Part model, mm, in its own coordinate system. A direction names the side the tool comes from. Round coordinates to 2 decimals unless told otherwise and drop trailing zeros. Order: outer loops, then holes, each group sorted by start corner. A loop starts at its lowest first (then second) coordinate and runs counter-clockwise, first axis right, second up. Notation, with made-up numbers: (66, 35) - (92, 35) arc R16 ccw to (92, 46) - close; hole circle Ø3 at (89, 71.5). An arc over 180 degrees is marked (long way). Answer as a JSON object with one key per item and string values.
```python
from build123d import *

# Parameters (mm, degrees)
SKETCH1_R           = 37.5
SKETCH1_R_2         = 27.5
BOSS_EXTRUDE1_DEPTH = 15
SKETCH2_R           = 32.5
SKETCH2_R_2         = 27.5
CUT_EXTRUDE1_DEPTH  = 7
SKETCH3_W           = 5
SKETCH3_H           = 40
CUT_EXTRUDE2_DEPTH  = 45
BOSS_EXTRUDE2_DEPTH = 45
SKETCH6_W           = 10
SKETCH6_H           = 40
CUT_EXTRUDE3_DEPTH  = 5
SKETCH7_W           = 10
SKETCH7_H           = 40
BOSS_EXTRUDE3_DEPTH = 12.5
SKETCH8_R           = 1.5
CUT_EXTRUDE4_DEPTH  = 10


with BuildPart() as part:
    # Sketch1 → Boss-Extrude1 (new body)
    # profile 1 of 2: a face of its own
    with BuildSketch(Plane.XY):
        Circle(SKETCH1_R)
        Circle(SKETCH1_R_2, mode=Mode.SUBTRACT)
    # profile 2 of 2: a face of its own
    with BuildSketch(Plane.XY):
        with BuildLine():
            Line((-23.101603537, -77.5), (21.898396463, -77.5))
            Line((21.898396463, -77.5), (21.898396463, -30.441915714))
            ThreePointArc((21.898396463, -30.441915714), (-0.752089542, -37.492457392), (-23.101603537, -29.5392267))
            Line((-23.101603537, -29.5392267), (-23.101603537, -77.5))
        make_face()
    extrude(amount=BOSS_EXTRUDE1_DEPTH)

    # Sketch2 → Cut-Extrude1 (cut)
    with BuildSketch(Plane(origin=(0, 0, 0), x_dir=(-1, 0, 0), z_dir=(0, 0, -1))):
        Circle(SKETCH2_R)
        Circle(SKETCH2_R_2, mode=Mode.SUBTRACT)
    extrude(amount=-CUT_EXTRUDE1_DEPTH, mode=Mode.SUBTRACT)

    # Sketch3 → Cut-Extrude2 (cut)
    with BuildSketch(Plane(origin=(21.898396463, 0, 0), x_dir=(0, 0, -1), z_dir=(1, 0, 0))):
        with Locations((-12.5, -57.5)):
            Rectangle(SKETCH3_W, SKETCH3_H)
    extrude(amount=-CUT_EXTRUDE2_DEPTH, mode=Mode.SUBTRACT)

    # Sketch5 → Boss-Extrude2 (add)
    with BuildSketch(Plane.ZY.offset(23.101603537)):
        Polygon((10, -37.5), (15, -37.5), (10, -77.5), align=None)
    extrude(amount=-BOSS_EXTRUDE2_DEPTH)

    # Sketch6 → Cut-Extrude3 (cut)
    with BuildSketch(Plane.XY.offset(15)):
        with Locations((-10.101603537, -57.5)):
            Rectangle(SKETCH6_W, SKETCH6_H)
        with Locations((8.898396463, -57.5)):
            Rectangle(SKETCH6_W, SKETCH6_H)
    extrude(amount=-CUT_EXTRUDE3_DEPTH, mode=Mode.SUBTRACT)

    # Sketch7 → Boss-Extrude3 (add)
    with BuildSketch(Plane(origin=(0, 0, 0), x_dir=(-1, 0, 0), z_dir=(0, 0, -1))):
        with Locations((-16.898396463, -57.5)):
            Rectangle(SKETCH7_W, SKETCH7_H)
        with Locations((18.101603537, -57.5)):
            Rectangle(SKETCH7_W, SKETCH7_H)
    extrude(amount=BOSS_EXTRUDE3_DEPTH)

    # Sketch8 → Cut-Extrude4 (cut)
    with BuildSketch(Plane.XY.offset(10)):
        with Locations((-9.101603537, -47.5)):
            Circle(SKETCH8_R)
        with Locations((-9.101603537, -67.5)):
            Circle(SKETCH8_R)
        with Locations((7.898396463, -67.5)):
            Circle(SKETCH8_R)
        with Locations((7.898396463, -47.5)):
            Circle(SKETCH8_R)
    extrude(amount=-CUT_EXTRUDE4_DEPTH, mode=Mode.SUBTRACT)


solid = part.part
```
Item 1: Cut at D-D (y = 23). Write the cut outline in (x, z).
Taken from the geometry:
{"outline": "(-29.62, 0) - (-22.96, 0) - (-22.96, 7) - (-15.07, 7) - (-15.07, 15) - (-29.62, 15) - close; (15.07, 7) - (22.96, 7) - (22.96, 0) - (29.62, 0) - (29.62, 15) - (15.07, 15) - close"}
Item 2: Cut at A-A (z = -1.5). Write the cut outline in (x, y), plus the area to 3 significant figures.
Taken from the geometry:
{"outline": "(-23.1, -77.5) - (-13.1, -77.5) - (-13.1, -37.5) - (-23.1, -37.5) - close; (11.9, -77.5) - (21.9, -77.5) - (21.9, -37.5) - (11.9, -37.5) - close", "area": "800 mm2"}
Item 3: Drop flat-ended pins along their axis: P1, Ø5, axis at x = -9.1, y = -67.5, coming from the +Z side; P2, Ø4, axis at y = 13, z = 3.5, coming from the +X side; P3, Ø3.5, axis at x = 7.9, y = -47.5, coming from the -Z side; P4, Ø1.8, axis at x = -9.1, y = -47.5, coming from the -Z side. Give the stop position or say it passes through.
Taken from the geometry:
{"P1": "z = 10", "P2": "x = 35.85", "P3": "z = 0", "P4": "through"}
Item 4: Probe L1, parallel to X at y = -67.5, z = 4.5; L2, parallel to Y at x = 0, z = 9.5; L3, parallel to X at y = -51, z = -0.25. List the from-to ranges inside material, lowest first. Write a range as from..to.
Taken from the geometry:
{"L1": "-23.1..-10.6, -7.6..6.4, 9.4..21.9", "L2": "-77.5..-27.5, 27.5..37.5", "L3": "-23.1..-13.1, 11.9..21.9"}
Item 5: Tool access for faces 5 (the flat face through (9, -37.5, 13)), 6 (the cylindrical face through (-5.961, -26.846, 10.944)), 7 (the flat face through (17, -37.5, -6)), 8 (the flat face through (21.898, -54, 1)), 9 (the flat face through (5, -28, 15)): list every direction of +Z, -Z, +X, -X, +Y, -Y with a clear straight run to the whole face (end or side of a thin tool).
Taken from the geometry:
{"face 5": "+Z, -Y", "face 6": "+Z, -Z", "face 7": "-Z, +X, -X, +Y", "face 8": "+Z, -Z, +X, -Y", "face 9": "+Z, +X, -X, +Y, -Y"}
Item 6: Two-plate mould, pull along X, no slides. Class faces 1 (the flat face through (13.898, -49, 11)), 2 (the flat face through (-0.665, -57.22, 12.535)), 3 (the flat face through (-23.102, -53, 1)), 4 (the cylindrical face through (2.063, 37.443, 7.395)): pulls with the +X half, pulls with the -X half, needs draft (parallel to the pull), parting line crosses it, or undercut.
Taken from the geometry:
{"face 1": "undercut", "face 2": "needs draft", "face 3": "pulls with the -X half", "face 4": "parting line crosses it"}
Item 7: Cut at B-B (x = 0). Write the cut outline in (y, z), plus the area to 3 significant figures.
Taken from the geometry:
{"outline": "(-77.5, 0) - (-32.5, 0) - (-32.5, 7) - (-27.5, 7) - (-27.5, 15) - (-37.5, 15) - (-77.5, 10) - close; (27.5, 7) - (32.5, 7) - (32.5, 0) - (37.5, 0) - (37.5, 15) - (27.5, 15) - close", "area": "730 mm2"}
Item 8: Cut at C-C (y = -67.5). Write the cut outline in (x, z).
Taken from the geometry:
{"outline": "(-23.1, -12.5) - (-13.1, -12.5) - (-13.1, 0) - (-10.6, 0) - (-10.6, 10) - (-15.1, 10) - (-15.1, 11.25) - (-23.1, 11.25) - close; (-7.6, 0) - (6.4, 0) - (6.4, 10) - (3.9, 10) - (3.9, 11.25) - (-5.1, 11.25) - (-5.1, 10) - (-7.6, 10) - close; (9.4, 0) - (11.9, 0) - (11.9, -12.5) - (21.9, -12.5) - (21.9, 11.25) - (13.9, 11.25) - (13.9, 10) - (9.4, 10) - close"}
